Check sheet for the modelled part. Datum: model origin and axes. Units: mm. A direction names the side the tool comes from. Round coordinates to 2 decimals unless told otherwise and drop trailing zeros. Write each loop counter-clockwise with the first axis right and the second up, starting at its lowest first coordinate (ties: lowest second). Pieces come first, ordered by that corner, then holes. Notation, with made-up numbers: M -24.5,12.5 L 30.5,12.5 A24 ccw 30.5,46.5 Z; hole C -24.75,17.5 d3. An arc over 180 degrees is marked long. Answer in a Markdown table with one row per item.
```python
from build123d import *

# Parameters (mm, degrees)
SKETCH3_W                     = 100
SKETCH3_H                     = 79
BOSS_EXTRUDE1_DEPTH           = 3.175
SKETCH5_W                     = 58.8
SKETCH5_H                     = 40
CUT_EXTRUDE2_DEPTH            = 3.175
SKETCH11_W                    = 6.35
SKETCH11_H                    = 3.175
BOSS_EXTRUDE2_DEPTH           = 3.175
LPATTERN2_COUNT               = 6
LPATTERN2_PITCH               = 6.35
LPATTERN2_COPY_1_SKETCH_W     = 6.35
LPATTERN2_COPY_1_SKETCH_H     = 3.175
LPATTERN2_COPY_1_DEPTH        = 3.175
LPATTERN2_COPY_2_SKETCH_W     = 6.35
LPATTERN2_COPY_2_SKETCH_H     = 3.175
LPATTERN2_COPY_2_DEPTH        = 3.175
LPATTERN2_COPY_3_SKETCH_W     = 6.35
LPATTERN2_COPY_3_SKETCH_H     = 3.175
LPATTERN2_COPY_3_DEPTH        = 3.175
LPATTERN2_COPY_4_SKETCH_W     = 6.35
LPATTERN2_COPY_4_SKETCH_H     = 3.175
LPATTERN2_COPY_4_DEPTH        = 3.175
LPATTERN2_COPY_5_SKETCH_W     = 6.35
LPATTERN2_COPY_5_SKETCH_H     = 3.175
LPATTERN2_COPY_5_DEPTH        = 3.175
LPATTERN2_COL_COUNT           = 6
LPATTERN2_COL_PITCH           = 6.35
LPATTERN2_COL_COPY_1_SKETCH_W = 6.35
LPATTERN2_COL_COPY_1_SKETCH_H = 3.175
LPATTERN2_COL_COPY_1_DEPTH    = 3.175
LPATTERN2_COL_COPY_2_SKETCH_W = 6.35
LPATTERN2_COL_COPY_2_SKETCH_H = 3.175
LPATTERN2_COL_COPY_2_DEPTH    = 3.175
LPATTERN2_COL_COPY_3_SKETCH_W = 6.35
LPATTERN2_COL_COPY_3_SKETCH_H = 3.175
LPATTERN2_COL_COPY_3_DEPTH    = 3.175
LPATTERN2_COL_COPY_4_SKETCH_W = 6.35
LPATTERN2_COL_COPY_4_SKETCH_H = 3.175
LPATTERN2_COL_COPY_4_DEPTH    = 3.175
LPATTERN2_COL_COPY_5_SKETCH_W = 6.35
LPATTERN2_COL_COPY_5_SKETCH_H = 3.175
LPATTERN2_COL_COPY_5_DEPTH    = 3.175
SKETCH13_W                    = 12.35
SKETCH13_H                    = 79
BOSS_EXTRUDE4_DEPTH           = 3.175
SKETCH14_W                    = 12.35
SKETCH14_H                    = 79
BOSS_EXTRUDE5_DEPTH           = 3.175
SKETCH15_R                    = 1.5
CUT_EXTRUDE4_DEPTH            = 10
SKETCH16_R                    = 1.5
CUT_EXTRUDE5_DEPTH            = 10


with BuildPart() as part:
    # Sketch3 → Boss-Extrude1 (new body)
    with BuildSketch(Plane(origin=(0, 0, 0), x_dir=(1, 0, 0), z_dir=(0, 1, 0))):
        with Locations((46, 22.5)):
            Rectangle(SKETCH3_W, SKETCH3_H)
    extrude(amount=BOSS_EXTRUDE1_DEPTH)

    # Sketch5 → Cut-Extrude2 (cut)
    with BuildSketch(Plane(origin=(0, 3.175, 0), x_dir=(1, 0, 0), z_dir=(0, 1, 0))):
        with Locations((44, 42)):
            Rectangle(SKETCH5_W, SKETCH5_H)
    extrude(amount=-CUT_EXTRUDE2_DEPTH, mode=Mode.SUBTRACT)

    # Sketch11 → Boss-Extrude2 (add)
    with BuildSketch(Plane(origin=(0, 3.175, 0), x_dir=(1, 0, 0), z_dir=(0, 1, 0))):
        with Locations((-4, 22.5)):
            Rectangle(SKETCH11_W, SKETCH11_H)
    boss_extrude2 = extrude(amount=-BOSS_EXTRUDE2_DEPTH)

    # Mirror2: Boss-Extrude2 across plane
    add(boss_extrude2.mirror(Plane.ZY.offset(-46)))

    # LPattern2: Boss-Extrude2 ×6
    with Locations(*[(0, 0, -i * LPATTERN2_PITCH) for i in range(1, LPATTERN2_COUNT)]):
        add(boss_extrude2)

    # LPattern2 copy 1 sketch → LPattern2 copy 1 (add)
    with BuildSketch(Plane(origin=(92, 3.175, -6.35), x_dir=(-1, 0, 0), z_dir=(0, 1, 0))):
        with Locations((-4, -22.5)):
            Rectangle(LPATTERN2_COPY_1_SKETCH_W, LPATTERN2_COPY_1_SKETCH_H)
    extrude(amount=-LPATTERN2_COPY_1_DEPTH)

    # LPattern2 copy 2 sketch → LPattern2 copy 2 (add)
    with BuildSketch(Plane(origin=(92, 3.175, -12.7), x_dir=(-1, 0, 0), z_dir=(0, 1, 0))):
        with Locations((-4, -22.5)):
            Rectangle(LPATTERN2_COPY_2_SKETCH_W, LPATTERN2_COPY_2_SKETCH_H)
    extrude(amount=-LPATTERN2_COPY_2_DEPTH)

    # LPattern2 copy 3 sketch → LPattern2 copy 3 (add)
    with BuildSketch(Plane(origin=(92, 3.175, -19.05), x_dir=(-1, 0, 0), z_dir=(0, 1, 0))):
        with Locations((-4, -22.5)):
            Rectangle(LPATTERN2_COPY_3_SKETCH_W, LPATTERN2_COPY_3_SKETCH_H)
    extrude(amount=-LPATTERN2_COPY_3_DEPTH)

    # LPattern2 copy 4 sketch → LPattern2 copy 4 (add)
    with BuildSketch(Plane(origin=(92, 3.175, -25.4), x_dir=(-1, 0, 0), z_dir=(0, 1, 0))):
        with Locations((-4, -22.5)):
            Rectangle(LPATTERN2_COPY_4_SKETCH_W, LPATTERN2_COPY_4_SKETCH_H)
    extrude(amount=-LPATTERN2_COPY_4_DEPTH)

    # LPattern2 copy 5 sketch → LPattern2 copy 5 (add)
    with BuildSketch(Plane(origin=(92, 3.175, -31.75), x_dir=(-1, 0, 0), z_dir=(0, 1, 0))):
        with Locations((-4, -22.5)):
            Rectangle(LPATTERN2_COPY_5_SKETCH_W, LPATTERN2_COPY_5_SKETCH_H)
    extrude(amount=-LPATTERN2_COPY_5_DEPTH)

    # LPattern2 col: Boss-Extrude2 ×6
    with Locations(*[(0, 0, i * LPATTERN2_COL_PITCH) for i in range(1, LPATTERN2_COL_COUNT)]):
        add(boss_extrude2)

    # LPattern2 col copy 1 sketch → LPattern2 col copy 1 (add)
    with BuildSketch(Plane(origin=(92, 3.175, 6.35), x_dir=(-1, 0, 0), z_dir=(0, 1, 0))):
        with Locations((-4, -22.5)):
            Rectangle(LPATTERN2_COL_COPY_1_SKETCH_W, LPATTERN2_COL_COPY_1_SKETCH_H)
    extrude(amount=-LPATTERN2_COL_COPY_1_DEPTH)

    # LPattern2 col copy 2 sketch → LPattern2 col copy 2 (add)
    with BuildSketch(Plane(origin=(92, 3.175, 12.7), x_dir=(-1, 0, 0), z_dir=(0, 1, 0))):
        with Locations((-4, -22.5)):
            Rectangle(LPATTERN2_COL_COPY_2_SKETCH_W, LPATTERN2_COL_COPY_2_SKETCH_H)
    extrude(amount=-LPATTERN2_COL_COPY_2_DEPTH)

    # LPattern2 col copy 3 sketch → LPattern2 col copy 3 (add)
    with BuildSketch(Plane(origin=(92, 3.175, 19.05), x_dir=(-1, 0, 0), z_dir=(0, 1, 0))):
        with Locations((-4, -22.5)):
            Rectangle(LPATTERN2_COL_COPY_3_SKETCH_W, LPATTERN2_COL_COPY_3_SKETCH_H)
    extrude(amount=-LPATTERN2_COL_COPY_3_DEPTH)

    # LPattern2 col copy 4 sketch → LPattern2 col copy 4 (add)
    with BuildSketch(Plane(origin=(92, 3.175, 25.4), x_dir=(-1, 0, 0), z_dir=(0, 1, 0))):
        with Locations((-4, -22.5)):
            Rectangle(LPATTERN2_COL_COPY_4_SKETCH_W, LPATTERN2_COL_COPY_4_SKETCH_H)
    extrude(amount=-LPATTERN2_COL_COPY_4_DEPTH)

    # LPattern2 col copy 5 sketch → LPattern2 col copy 5 (add)
    with BuildSketch(Plane(origin=(92, 3.175, 31.75), x_dir=(-1, 0, 0), z_dir=(0, 1, 0))):
        with Locations((-4, -22.5)):
            Rectangle(LPATTERN2_COL_COPY_5_SKETCH_W, LPATTERN2_COL_COPY_5_SKETCH_H)
    extrude(amount=-LPATTERN2_COL_COPY_5_DEPTH)

    # Sketch13 → Boss-Extrude4 (add)
    with BuildSketch(Plane(origin=(0, 3.175, 0), x_dir=(1, 0, 0), z_dir=(0, 1, 0))):
        with Locations((-13.35, 22.5)):
            Rectangle(SKETCH13_W, SKETCH13_H)
    extrude(amount=-BOSS_EXTRUDE4_DEPTH)

    # Sketch14 → Boss-Extrude5 (add)
    with BuildSketch(Plane(origin=(0, 3.175, 0), x_dir=(1, 0, 0), z_dir=(0, 1, 0))):
        with Locations((105.35, 22.5)):
            Rectangle(SKETCH14_W, SKETCH14_H)
    extrude(amount=-BOSS_EXTRUDE5_DEPTH)

    # Sketch15 → Cut-Extrude4 (cut)
    with BuildSketch(Plane(origin=(0, 3.175, 0), x_dir=(1, 0, 0), z_dir=(0, 1, 0))):
        with Locations(Location((-13.35, 54, 0), (0, 0, 270))):
            Circle(SKETCH15_R)
        with Locations(Location((-13.35, -9, 0), (0, 0, 270))):
            Circle(SKETCH15_R)
    extrude(amount=-CUT_EXTRUDE4_DEPTH, mode=Mode.SUBTRACT)

    # Sketch16 → Cut-Extrude5 (cut)
    with BuildSketch(Plane(origin=(0, 3.175, 0), x_dir=(1, 0, 0), z_dir=(0, 1, 0))):
        with Locations(Location((105.35, 54, 0), (0, 0, 270))):
            Circle(SKETCH16_R)
        with Locations(Location((105.35, -9, 0), (0, 0, 270))):
            Circle(SKETCH16_R)
    extrude(amount=-CUT_EXTRUDE5_DEPTH, mode=Mode.SUBTRACT)


solid = part.part
```
1. Section check D-D, the plane y = 2.05. Count the separate pieces of the cut face and the enclosed holes in it, and give its area (3 significant figures).
Found:
| item | result |
|---|---|
| separate pieces | 1 |
| enclosed holes | 24 |
| area | 7,690 mm2 |
2. Scan lines: L1, parallel to Z at x = 105.35, y = 1.1; L2, parallel to X at y = 0.8, z = 9 (3 decimals); L3, parallel to X at y = 2.55, z = -54 (3 decimals). Record each from-to range of solid material in increasing order.
Found:
| item | result |
|---|---|
| L1 | z = -62 to -55.5, -52.5 to 7.5, 10.5 to 17 |
| L2 | x = -19.525 to -14.85, -11.85 to 103.85, 106.85 to 111.525 |
| L3 | x = -19.525 to -14.85, -11.85 to 14.6, 73.4 to 103.85, 106.85 to 111.525 |
3. Section check B-B, the plane x = -13.35. Record the cut outline in (y, z) (3 decimals), and give its area (3 significant figures).
Found:
| item | result |
|---|---|
| outline | M 0,-62 L 3.175,-62 L 3.175,-55.5 L 0,-55.5 Z; M 0,-52.5 L 3.175,-52.5 L 3.175,7.5 L 0,7.5 Z; M 0,10.5 L 3.175,10.5 L 3.175,17 L 0,17 Z |
| area | 232 mm2 |
4. Go/stop test with flat-tipped pins: pin 1 (1 mm diameter, centred on x = 98, y = 2, fed in from +Z); pin 2 (1.6 mm diameter, centred on x = -5.5, y = 1, fed in from -Z). Record where each tip stops, or that it passes through.
Found:
| item | result |
|---|---|
| pin 1 | stops at z = 10.84 |
| pin 2 | stops at z = -55.84 |
5. Access from +Z, -Z, +X, -X, +Y, -Y to the whole of each face (thin tool, end or side, straight path). Record for faces 3 (the face through (-6, 2, -27.263)), 4 (the face through (-7.175, 2, -59)), 5 (the face through (96, 2, 14)).
Found:
| item | result |
|---|---|
| face 3 | +Y, -Y |
| face 4 | -Z, +Y, -Y |
| face 5 | +Z, +Y, -Y |
6. Section check C-C, the plane z = -19. Record the cut outline in (x, y) (3 decimals), and give its area (3 significant figures).
Found:
| item | result |
|---|---|
| outline | M -19.525,0 L -7.175,0 L -7.175,3.175 L -19.525,3.175 Z; M -4,0 L 96,0 L 96,3.175 L -4,3.175 Z; M 99.175,0 L 111.525,0 L 111.525,3.175 L 99.175,3.175 Z |
| area | 396 mm2 |
7. Draft check along X on faces 1 (the face through (98, 2, 7.662)), 2 (the face through (85, 2, -62)). Enter one of: +X half, -X half, draft (parallel to the pull), parting line (faces both ways), or undercut.
Found:
| item | result |
|---|---|
| face 1 | undercut |
| face 2 | draft |
8. Section check A-A, the plane z = -54. Record the cut outline in (x, y) (3 decimals), and give its area (3 significant figures).
Found:
| item | result |
|---|---|
| outline | M -19.525,0 L -14.85,0 L -14.85,3.175 L -19.525,3.175 Z; M -11.85,0 L 14.6,0 L 14.6,3.175 L -11.85,3.175 Z; M 73.4,0 L 103.85,0 L 103.85,3.175 L 73.4,3.175 Z; M 106.85,0 L 111.525,0 L 111.525,3.175 L 106.85,3.175 Z |
| area | 210 mm2 |
